```python
from build123d import *

# Parameters (mm, degrees)
SKETCH_1_R      = 15
SKETCH_1_R_2    = 2.1
SKETCH_1_R_3    = 1.5
EXTRUDE_1_DEPTH = 3
FILLET_2_R      = 2
FILLET_3_R      = 10


with BuildPart() as part:
    # 草图1 → 凸台-拉伸1 (new body)
    with BuildSketch(Plane(origin=(0, 0, 0), x_dir=(0, 0, -1), z_dir=(1, 0, 0))):
        with BuildLine():
            Line((-32.4, 72.5), (32.4, 72.5))
            Line((32.4, 72.5), (32.4, 57.5))
            Line((32.4, 57.5), (25, 44.682824024))
            Line((25, 44.682824024), (25, 0))
            ThreePointArc((25, 0), (0, -25), (-25, 0))
            Line((-25, 0), (-25, 44.682824024))
            Line((-25, 44.682824024), (-32.4, 57.5))
            Line((-32.4, 57.5), (-32.4, 72.5))
        make_face()
        Circle(SKETCH_1_R, mode=Mode.SUBTRACT)
        with Locations((0, 20)):
            Circle(SKETCH_1_R_2, mode=Mode.SUBTRACT)
        with Locations((17.320508076, -10)):
            Circle(SKETCH_1_R_2, mode=Mode.SUBTRACT)
        with Locations((-17.320508076, -10)):
            Circle(SKETCH_1_R_2, mode=Mode.SUBTRACT)
        with Locations((-25, 65)):
            Circle(SKETCH_1_R_3, mode=Mode.SUBTRACT)
        with Locations((0, 65)):
            Circle(SKETCH_1_R_3, mode=Mode.SUBTRACT)
        with Locations((25, 65)):
            Circle(SKETCH_1_R_3, mode=Mode.SUBTRACT)
        with BuildLine():
            Line((-19, 57.5), (-4, 57.5))
            Line((-4, 57.5), (-4, 27.5))
            Line((-4, 27.5), (-12, 27.5))
            ThreePointArc((-12, 27.5), (-13.829211823, 42.889850575), (-19, 57.5))
        make_face(mode=Mode.SUBTRACT)
        with BuildLine():
            Line((4, 27.5), (12, 27.5))
            ThreePointArc((12, 27.5), (13.829211823, 42.889850575), (19, 57.5))
            Line((19, 57.5), (4, 57.5))
            Line((4, 57.5), (4, 27.5))
        make_face(mode=Mode.SUBTRACT)
    extrude(amount=EXTRUDE_1_DEPTH)

    # 圆角2
    fillet_2_edges = [part.edges().sort_by_distance(p)[0] for p in [
        (1.5, 72.5, 32.4),
        (1.5, 72.5, -32.4),
        (1.5, 57.5, -32.4),
        (1.5, 57.5, 32.4),
        (1.5, 57.5, 19),
        (1.5, 27.5, 12),
        (1.5, 27.5, 4),
        (1.5, 57.5, 4),
        (1.5, 27.5, -12),
        (1.5, 57.5, -19),
        (1.5, 57.5, -4),
        (1.5, 27.5, -4),
    ]]
    fillet(fillet_2_edges, radius=FILLET_2_R)

    # 圆角3
    fillet_3_edges = [part.edges().sort_by_distance(p)[0] for p in [
        (1.5, 44.682824024, -25),
        (1.5, 44.682824024, 25),
    ]]
    fillet(fillet_3_edges, radius=FILLET_3_R)


solid = part.part
```
Source: CAD feature listing. Evaluate the final solid. Frame: model axes, mm. A direction names the side the tool comes from. Give positions to 0.01 mm unless a question says otherwise; leave off trailing zeros. Order: outer loops, then holes, each group sorted by start corner. A loop starts at its lowest first (then second) coordinate and runs counter-clockwise, first axis right, second up.
(1) Pull-direction query (Z, two-part tool) for faces 1 (the face through (1.48, 21.77, -1.13)), 2 (the face through (1.479, 52.09, -29.276)), 3 (the face through (1.52, 44.63, 25.35)); classes: +Z half, -Z half, draft (parallel to the pull), parting line (faces both ways), or undercut.
(2) Section query B-B (y = 41). Return the cut outline in (x, z), plus the area to 3 significant figures.
(3) Contact query for flat-ended pins moving along their axis: P1, Ø2.5, axis at y = 20, z = 0, coming from the +X side; P2, Ø1.5, axis at x = 1, z = -13.5, coming from the -Y side. Output: stop coordinate, or through.
(4) Material intervals for line 1 along Y through (x, z) = (2.2, 0); line 2 along Z through (x, y) = (2.6, 65); line 3 along Y through (x, z) = (2.05, -8.5), sorted ascending.
(5) Section query C-C (z = 14). Return the cut outline in (x, y), plus the area to 3 significant figures.
(6) Section query D-D (y = 65). Return the cut outline in (x, z), plus the area to 3 significant figures.
(7) Access query for faces 4 (the face through (1.52, 28.08, 11.45)), 5 (the face through (1.479, -24.994, -0.55)). Directions: +Z, -Z, +X, -X, +Y, -Y. A direction counts if a zero-diameter tool reaches every point of the face in a straight line with its end or side. Return the directions, or none.
(8) Section query A-A (y = 20). Return the cut outline in (x, z), plus the area to 3 significant figures.
Outcome:
1. face 1: undercut
1. face 2: -Z half
1. face 3: +Z half
2. outline: (0, -25) - (3, -25) - (3, -13.42) - (0, -13.42) - close; (0, -4) - (3, -4) - (3, 4) - (0, 4) - close; (0, 13.42) - (3, 13.42) - (3, 25) - (0, 25) - close
2. area: 93.5 mm2
3. P1: passes through
3. P2: stops at y = -21.5
4. line 1: y = -25 to -15, 15 to 17.9, 22.1 to 63.5, 66.5 to 72.5
4. line 2: z = -32.4 to -26.5, -23.5 to -1.5, 1.5 to 23.5, 26.5 to 32.4
4. line 3: y = -23.51 to -12.36, 12.36 to 27.5, 57.5 to 72.5
5. outline: (0, -20.71) - (3, -20.71) - (3, -5.39) - (0, -5.39) - close; (0, 5.39) - (3, 5.39) - (3, 43.6) - (0, 43.6) - close; (0, 57.5) - (3, 57.5) - (3, 72.5) - (0, 72.5) - close
5. area: 206 mm2
6. outline: (0, -32.4) - (3, -32.4) - (3, -26.5) - (0, -26.5) - close; (0, -23.5) - (3, -23.5) - (3, -1.5) - (0, -1.5) - close; (0, 1.5) - (3, 1.5) - (3, 23.5) - (0, 23.5) - close; (0, 26.5) - (3, 26.5) - (3, 32.4) - (0, 32.4) - close
6. area: 167 mm2
7. face 4: +X, -X
7. face 5: +X, -X, -Y
8. outline: (0, -25) - (3, -25) - (3, -2.1) - (0, -2.1) - close; (0, 2.1) - (3, 2.1) - (3, 25) - (0, 25) - close
8. area: 137 mm2
